```python
from build123d import *

# Parameters (mm, degrees)
EXTRUDE_1_DEPTH     = 2
SKETCH_2_W          = 45.974
SKETCH_2_H          = 20
SKETCH_2_H_2        = 15
CUT_EXTRUDE_1_DEPTH = 10


with BuildPart() as part:
    # Эскиз1 → Бобышка-Вытянуть1 (new body)
    with BuildSketch(Plane.XY):
        Polygon((0, -61.595), (0, -104.902), (-45.974, -104.902), (-45.974, -61.595), (-48.006, -61.595), (-48.006, -51.689), (-45.974, -51.689), (-45.974, 0), (0, 0), (0, -51.689), (2.032, -51.689), (2.032, -61.595), align=None)
    extrude(amount=EXTRUDE_1_DEPTH)

    # Эскиз2 → Вырез-Вытянуть1 (cut)
    with BuildSketch(Plane(origin=(0, 0, 0), x_dir=(-1, 0, 0), z_dir=(0, 0, -1))):
        with Locations((22.987, -10)):
            Rectangle(SKETCH_2_W, SKETCH_2_H)
        with Locations((22.987, -97.402)):
            Rectangle(SKETCH_2_W, SKETCH_2_H_2)
    extrude(amount=-CUT_EXTRUDE_1_DEPTH, mode=Mode.SUBTRACT)


solid = part.part
```
For this review, take the finished solid that the model builds, in its own axes (mm). A direction names the side the tool comes from. Coordinates: 2 decimals unless noted, no trailing zeros. Loops run counter-clockwise (first coordinate to the right, second up) from the corner with the lowest first, then second, coordinate; pieces in that order, holes last. Notation, with made-up numbers: (32, 6) -> (83, 6) arc R22 ccw to (83, 30) -> close; hole circle Ø10 at (62, -23.5). An arc over 180 degrees is marked (long way). Return JSON: item names as keys, results as strings. Group by question number.
(1) To check wall thickness, follow L1, parallel to X at y = -81, z = 1.05. State the ranges of the line that lie inside material, in increasing order.
(2) Consider section A-A, the plane z = 1.6. Give the boundary of the cut face in (x, y) (3 decimals), plus the area to 3 significant figures.
(3) Tool access review of faces 1 (the flat face through (-45.974, -36, 1)), 2 (the flat face through (0, -76, 1)), 3 (the flat face through (-47, -61.595, 1)): name each direction out of +Z, -Z, +X, -X, +Y, -Y from which nothing blocks a thin tool from reaching the whole face with its end or side.
(4) Consider section B-B, the plane y = -33.5. Give the boundary of the cut face in (x, z).
(5) For pin 1 Ø1 at (x, z) = (1, 1) entering from -Y (3 decimals); pin 2 Ø1 at (y, z) = (-30.5, 1) entering from +X; pin 3 Ø3 at (x, y) = (-23.5, -66.5) entering from -Z; pin 4 Ø0.6 at (y, z) = (-32.5, 1) entering from -X, all flat-tipped, find the tip position at first contact; note any pin that passes through.
Results below:
{
 "1": {"L1": "x = -45.97 to 0"},
 "2": {"outline": "(-48.006, -61.595) -> (-45.974, -61.595) -> (-45.974, -89.902) -> (0, -89.902) -> (0, -61.595) -> (2.032, -61.595) -> (2.032, -51.689) -> (0, -51.689) -> (0, -20) -> (-45.974, -20) -> (-45.974, -51.689) -> (-48.006, -51.689) -> close", "area": "3,250 mm2"},
 "3": {"face 1": "+Z, -Z, -X, +Y", "face 2": "+Z, -Z, +X, -Y", "face 3": "+Z, -Z, -X, -Y"},
 "4": {"outline": "(-45.97, 0) -> (0, 0) -> (0, 2) -> (-45.97, 2) -> close"},
 "5": {"pin 1": "stops at y = -61.595", "pin 2": "stops at x = 0", "pin 3": "stops at z = 0", "pin 4": "stops at x = -45.97"}
}
